Work out the finished part from the listing and answer in its coordinate system (mm). A direction names the side the tool comes from. Coordinates: 2 decimals unless noted, no trailing zeros. Order: outer loops, then holes, each group sorted by start corner. A loop starts at its lowest first (then second) coordinate and runs counter-clockwise, first axis right, second up. Notation, with made-up numbers: M -17.5,69 L 10.5,69 A24 ccw 10.5,102 Z; hole C 62.25,12 d10. An arc over 180 degrees is marked long. Use a Markdown table: item, result.
Autodesk Inventor part; units mm, degrees
ref_plane "YZ Plane" through (0, 0, 0) normal (1, 0, 0) x (0, 1, 0)
ref_plane "XZ Plane" through (0, 0, 0) normal (0, 1, 0) x (-1, 0, 0)
ref_plane "XY Plane" through (0, 0, 0) normal (0, 0, 1) x (1, 0, 0)
sketch "Sketch1" plane through (0, 0, 0) normal (0, 1, 0) x (-1, 0, 0)
  circle A0 centre (0, 0) radius 4.8006
  circle A1 centre (0, 0) radius 6.3881
  dimension "d0" = 9.6012
  dimension "d1" = 1.5875
extrude "Extrusion1" add sketch "Sketch1" along normal blind 19.05
extrude "Extrusion2" add sketch "Sketch1" along normal blind 3.175 contours A0
fillet "Fillet1" radius 1.5875 1 edges at (6.3881, 0, 0)
chamfer "Chamfer1" distance 0.7937 angle 45 1 edges at (4.8006, 19.05, 0)
fillet "Fillet2" radius 1.5875 1 edges at (4.8006, 18.2563, 0)
properties part number "137 V Dipole Cap"
(1) Given P1, Ø5, axis at y = 8.5, z = -3.5, coming from the -X side; P2, Ø4, axis at x = 3.5, y = 13.5, coming from the -Z side, each flat-ended and moving along its own axis, determine where each tip first touches the part or whether it passes through.
Conclusion:
| item | result |
|---|---|
| P1 | x = -6.31 |
| P2 | z = -6.21 |
(2) Determine the mould class of faces 3 (the cylindrical face through (-4.58, 10.29, -1.44)), 4 (the flat face through (0, 0, 0)), 5 (the cylindrical face through (-6.1, 10.2, -1.9)) for opening direction X: pulls with the +X half, pulls with the -X half, needs draft (parallel to the pull), parting line crosses it, or undercut.
Conclusion:
| item | result |
|---|---|
| face 3 | undercut |
| face 4 | needs draft |
| face 5 | parting line crosses it |
(3) Which of the six approach directions +Z, -Z, +X, -X, +Y, -Y give full straight-line access (tool end or side, diameter ignored) to faces 1 (the flat face through (0, 19.05, -6)), 2 (the flat face through (0, 3.175, 0))?
Conclusion:
| item | result |
|---|---|
| face 1 | +Z, -Z, +X, -X, +Y |
| face 2 | +Y |
(4) A cutting plane is placed at A-A (y = 2.5). Determine the outline of the cut face in (x, z).
Conclusion:
| item | result |
|---|---|
| outline | C 0,0 d12.78 |
(5) A cutting plane is placed at B-B (y = 12.75). Determine the outline of the cut face in (x, z).
Conclusion:
| item | result |
|---|---|
| outline | C 0,0 d12.78; hole C 0,0 d9.6 |
(6) Straight lines are drawn through the part: L1, parallel to Z at x = 0, y = 11.5; L2, parallel to X at y = 10.25, z = -1.25 (3 decimals); L3, parallel to Z at x = 3.5, y = 9.75. For each, find the intervals that lie inside material, in ascending order.
Conclusion:
| item | result |
|---|---|
| L1 | -6.39 to -4.8, 4.8 to 6.39 |
| L2 | -6.265 to -4.635, 4.635 to 6.265 |
| L3 | -5.34 to -3.29, 3.29 to 5.34 |
